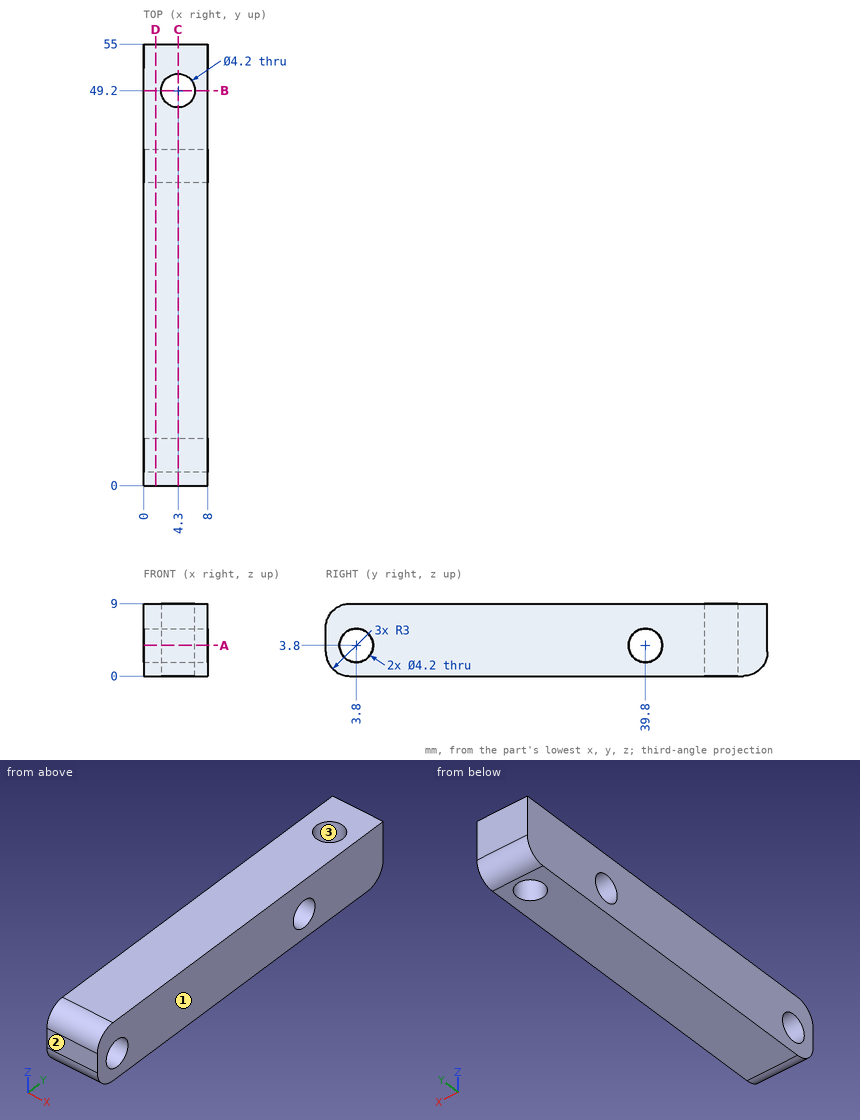
Geometry check sheet. Reference: drawing and pictorial views, mm from the part's lowest x, y, z. Give positions to 0.01 mm unless a question says otherwise; leave off trailing zeros. Order: outer loops, then holes, each group sorted by start corner. A loop starts at its lowest first (then second) coordinate and runs counter-clockwise, first axis right, second up. Notation, with made-up numbers: (20, 16.25) -> (52, 16.25) arc R23 cw to (52, 47.25) -> close; hole circle Ø10 at (-22.75, 77.5). An arc over 180 degrees is marked (long way). Use CSV: the item, a comma, the result in double quotes. Start each with the question number.
1) Sectioned sample at D-D, the plane x = 1.5. Record the boundary of the cut face in (y, z), plus the area to 3 significant figures.
2) Mould release check, pull along Y, two halves, no side actions. Record for the marked faces 1, 2 and 3: released by +Y, released by -Y, zero draft, split by the parting line, or undercut.
3) Sectioned sample at A-A, the plane z = 3.8. Record the boundary of the cut face in (x, y), plus the area to 3 significant figures.
4) Go/stop test with a flat-tipped pin: P1, Ø4, axis at y = 3.8, z = 3.8, coming from the -X side. Record where the tip stops, or that it passes through.
5) Material ranges on line 1 (Y direction, x = 6.75, z = 3.75); line 2 (X direction, y = 49.2, z = 6.25); line 3 (Z direction, x = 2.5, y = 3.8), recorded low to high. Write a range as from..to.
6) Sectioned sample at B-B, the plane y = 49.2. Record the boundary of the cut face in (x, z).
7) Sectioned sample at C-C, the plane x = 4.3. Record the boundary of the cut face in (y, z), plus the area to 3 significant figures.
Recorded:
1,outline,"(0, 3) arc R3 ccw to (3, 0) -> (52, 0) arc R3 ccw to (55, 3) -> (55, 9) -> (3, 9) arc R3 ccw to (0, 6) -> close; hole circle Ø4.2 at (3.8, 3.8); hole circle Ø4.2 at (39.8, 3.8)"
1,area,"461 mm2"
2,face 1,"zero draft"
2,face 2,"released by -Y"
2,face 3,"undercut"
3,outline,"(0, 0) -> (8, 0) -> (8, 1.7) -> (0, 1.7) -> close; (0, 5.9) -> (8, 5.9) -> (8, 37.7) -> (0, 37.7) -> close; (0, 41.9) -> (8, 41.9) -> (8, 55) -> (0, 55) -> close; hole circle Ø4.2 at (4.3, 49.2)"
3,area,"359 mm2"
4,P1,"through"
5,line 1,"0..1.7, 5.9..37.7, 41.9..55"
5,line 2,"0..2.2, 6.4..8"
5,line 3,"0..1.7, 5.9..9"
6,outline,"(0, 0) -> (2.2, 0) -> (2.2, 9) -> (0, 9) -> close; (6.4, 0) -> (8, 0) -> (8, 9) -> (6.4, 9) -> close"
7,outline,"(0, 3) arc R3 ccw to (3, 0) -> (47.1, 0) -> (47.1, 9) -> (3, 9) arc R3 ccw to (0, 6) -> close; (51.3, 0) -> (52, 0) arc R3 ccw to (55, 3) -> (55, 9) -> (51.3, 9) -> close; hole circle Ø4.2 at (3.8, 3.8); hole circle Ø4.2 at (39.8, 3.8)"
7,area,"424 mm2"
